Can you work these out from the model? Positions are in its coordinate system, mm. Give positions to 0.01 mm unless a question says otherwise; leave off trailing zeros. Loops run counter-clockwise (first coordinate to the right, second up) from the corner with the lowest first, then second, coordinate; pieces in that order, holes last. Notation, with made-up numbers: M 51.25,14 L 77.25,14 A12 ccw 77.25,26 Z; hole C 12,-5 d9. An arc over 180 degrees is marked long. Use CSV: the item, a comma, the result in double quotes.
Autodesk Inventor part; units mm, degrees
ref_plane "YZ Plane" through (0, 0, 0) normal (1, 0, 0) x (0, 1, 0)
ref_plane "XZ Plane" through (0, 0, 0) normal (0, 1, 0) x (-1, 0, 0)
ref_plane "XY Plane" through (0, 0, 0) normal (0, 0, 1) x (1, 0, 0)
sketch "Sketch1" plane through (0, 0, 0) normal (0, 0, 1) x (1, 0, 0)
  line L0 (151.725, 24) -> (151.725, -206)
  line L1 (151.725, -206) -> (-41.7, -206)
  line L2 (-41.7, -206) -> (-41.7, 24)
  line L3 (151.725, 24) -> (103.3, 44)
  line L4 (3.3, 44) -> (-41.7, 24)
  line L5 (78.3, 44) -> (78.3, -16)
  line L6 (3.3, 44) -> (18.3, 44)
  line L7 (78.3, 44) -> (103.3, 44)
  line L8 (-34.2, -33.5) -> (-34.2, 11.5)
  line L9 (-2.95, 11.5) -> (-2.95, -33.5)
  line L10 (-36.7, -41) -> (-0.45, -41)
  line L11 (-0.45, -41) -> (-0.45, 19)
  line L12 (-0.45, 19) -> (-36.7, 19)
  line L13 (-36.7, 19) -> (-36.7, -41)
  line L14 (110.475, -41) -> (146.725, -41)
  line L15 (146.725, -41) -> (146.725, 19)
  line L16 (146.725, 19) -> (110.475, 19)
  line L17 (110.475, 19) -> (110.475, -41)
  line L18 (110.475, -191) -> (146.725, -191)
  line L19 (146.725, -191) -> (146.725, -131)
  line L20 (146.725, -131) -> (110.475, -131)
  line L21 (110.475, -131) -> (110.475, -191)
  line L22 (-36.7, -191) -> (-0.45, -191)
  line L23 (-0.45, -191) -> (-0.45, -131)
  line L24 (-0.45, -131) -> (-36.7, -131)
  line L25 (-36.7, -131) -> (-36.7, -191)
  line L26 (144.225, -33.5) -> (144.225, 11.5)
  line L27 (112.975, 11.5) -> (112.975, -33.5)
  line L28 (112.975, -183.5) -> (112.975, -138.5)
  line L29 (144.225, -138.5) -> (144.225, -183.5)
  line L30 (-34.2, -138.5) -> (-34.2, -183.5)
  line L31 (-2.95, -183.5) -> (-2.95, -138.5)
  line L32 (75.3, -16) -> (75.2995, -26)
  line L33 (75.2995, -26) -> (78.2995, -26)
  line L34 (78.2995, -26) -> (78.3, -16)
  line L35 (65.3, -16) -> (65.2995, -26)
  line L36 (65.2995, -26) -> (68.2995, -26)
  line L37 (68.2995, -26) -> (68.3, -16)
  line L38 (55.3, -16) -> (55.2995, -26.1226)
  line L39 (55.2995, -26.1226) -> (58.2995, -26.1227)
  line L40 (58.2995, -26.1227) -> (58.3, -16)
  line L41 (78.3, -16) -> (78.3, -16)
  line L42 (75.3, -16) -> (68.3, -16)
  line L43 (65.3, -16) -> (58.3, -16)
  line L44 (45.3, -16) -> (45.2995, -25.9999)
  line L45 (48.2995, -26) -> (48.3, -16)
  line L46 (45.2995, -25.9999) -> (48.2995, -26)
  line L47 (55.3, -16) -> (48.3, -16)
  line L48 (38.2995, -26) -> (38.3, -16)
  line L49 (35.2995, -26) -> (38.2995, -26)
  line L50 (35.3, -16) -> (35.2995, -26)
  line L51 (28.2995, -26) -> (28.3, -16)
  line L52 (25.2995, -26) -> (28.2995, -26)
  line L53 (25.3, -16) -> (25.2995, -26)
  line L54 (45.3, -16) -> (38.3, -16)
  line L55 (35.3, -16) -> (28.3, -16)
  line L56 (18.3, 44) -> (25.3, 44)
  line L57 (25.3, 44) -> (25.3, -16)
  point P0 (-34.2, -11)
  point P1 (-36.7, -11)
  point P2 (128.6, -41)
  point P3 (110.475, -11)
  point P4 (112.975, -11)
  point P5 (128.6, -191)
  point P6 (128.6, -131)
  point P7 (110.475, -161)
  point P8 (112.975, -161)
  point P9 (-36.7, -161)
  point P10 (-34.2, -161)
  point P11 (75.2998, -21)
  point P12 (78.2998, -21)
  point P13 (76.775, -16.5)
  point P14 (76.7995, -26)
  point P15 (65.2998, -21)
  point P16 (68.2998, -21)
  point P17 (66.775, -16.5)
  point P18 (66.7995, -26)
  point P19 (55.2998, -21.0613)
  point P20 (58.2998, -21.0613)
  point P21 (56.775, -16.5)
  point P22 (56.7995, -26.1226)
  point P23 (45.2998, -20.9999)
  point P24 (46.7995, -25.9999)
  point P25 (43.0984, -16.3775)
  point P26 (48.2998, -21)
  point P27 (38.2998, -21)
  point P28 (36.7995, -26)
  point P29 (35.2998, -21)
  point P30 (28.2998, -21)
  point P31 (26.7995, -26)
  point P32 (25.2998, -21)
  point P33 (21.8, -16)
  point P34 (78.3, -16)
  point P35 (51.8, -16)
  point P36 (71.8, -16)
  dimension "d19" = 20
  dimension "d21" = 20
  dimension "d23" = 100
  dimension "d26" = 60
  dimension "d29" = 250
  dimension "d32" = 2.5
  dimension "d33" = 2.5
  dimension "d34" = 60
  dimension "d35" = 0
  dimension "d36" = 5
  dimension "d37" = 25
  dimension "d39" = 2.5
  dimension "d40" = 2.5
  dimension "d41" = 5
  dimension "d43" = 60
  dimension "d44" = 0
  dimension "d45" = 60
  dimension "d46" = 2.5
  dimension "d47" = 0
  dimension "d48" = 2.5
  dimension "d49" = 2.5
  dimension "d50" = 2.5
  dimension "d51" = 60
  dimension "d52" = 0
  dimension "d55" = 250
  dimension "d75" = 3
  dimension "d76" = 10
  dimension "d77" = 7
  dimension "d79" = 3
  dimension "d80" = 10
  dimension "d81" = 3
  dimension "d82" = 10
  dimension "d84" = 7
  dimension "d86" = 7
  dimension "d87" = 7
  dimension "d88" = 3
  dimension "d89" = 3
  dimension "d90" = 3
  dimension "d92" = 7
  dimension "d93" = 45
  dimension "d95" = 90
  dimension "d98" = 10
  dimension "d100" = 10
  dimension "d101" = 10
  dimension "d102" = 10
  dimension "d103" = 60
  dimension "d104" = 60
  dimension "d105" = 60
  dimension "d106" = 60
  dimension "d108" = 0
  dimension "d112" = 22
  dimension "d113" = 53
extrude "Extrusion2" add sketch "Sketch1" along normal blind 3
properties part number "car platform"
Q1. I want a section at B-B, the plane x = 132. Please give me the cut outline in (y, z), then the cut area to 3 significant figures.
Model answer:
outline,"M -206,0 L -191,0 L -191,3 L -206,3 Z; M -131,0 L -41,0 L -41,3 L -131,3 Z; M 19,0 L 32.15,0 L 32.15,3 L 19,3 Z"
area,"354 mm2"
Q2. I'm going to push flat-ended pins straight in: P1, Ø0.9, axis at x = 71, z = 1, coming from the +Y side; P2, Ø1.5, axis at x = -21, z = 2, coming from the +Y side. Where does each tip first touch, or does it pass through?
Model answer:
P1,"y = -16"
P2,"y = 33.53"
Q3. I want a section at C-C, the plane z = 1.7. State how many separate pieces and enclosed holes the cut face has, then the cut area to 3 significant figures.
Model answer:
separate pieces,"1"
enclosed holes,"4"
area,"35,400 mm2"
Q4. I want a section at D-D, the plane x = -10. Please give me the cut outline in (y, z).
Model answer:
outline,"M -206,0 L -191,0 L -191,3 L -206,3 Z; M -131,0 L -41,0 L -41,3 L -131,3 Z; M 19,0 L 38.09,0 L 38.09,3 L 19,3 Z"
Q5. I want a section at A-A, the plane y = 6.5. Please give me the cut outline in (x, z) (3 decimals).
Model answer:
outline,"M -41.7,0 L -36.7,0 L -36.7,3 L -41.7,3 Z; M -0.45,0 L 25.3,0 L 25.3,3 L -0.45,3 Z; M 78.3,0 L 110.475,0 L 110.475,3 L 78.3,3 Z; M 146.725,0 L 151.725,0 L 151.725,3 L 146.725,3 Z"
Q6. Please list where these lines run through material, in increasing order: L1, parallel to X at y = -174, z = 0.5 (3 decimals); L2, parallel to X at y = 3, z = 1.5 (3 decimals); L3, parallel to Y at x = -18.5, z = 0.25. Write a range as from..to.
Model answer:
L1,"-41.7..-36.7, -0.45..110.475, 146.725..151.725"
L2,"-41.7..-36.7, -0.45..25.3, 78.3..110.475, 146.725..151.725"
L3,"-206..-191, -131..-41, 19..34.31"
